from build123d import *

# Parameters (mm, degrees)
SKETCH_R           = 3.5
PAD_DEPTH          = 4
SKETCH001_W        = 5
SKETCH001_H        = 3.5
PAD001_DEPTH       = 17
POLARPATTERN_COUNT = 4
PAD002_DEPTH       = 17
PAD004_DEPTH       = 4
PAD005_DEPTH       = 20


with BuildPart() as part:
    # Sketch → Pad (new body)
    with BuildSketch(Plane.XY):
        Polygon((-9.8, 2.5), (-9.8, -2.5), (-2.5, -9.8), (2.5, -9.8), (9.8, -2.5), (9.8, 2.5), (2.5, 9.8), (-2.5, 9.8), align=None)
        Circle(SKETCH_R, mode=Mode.SUBTRACT)
    extrude(amount=-PAD_DEPTH)

    # Sketch001 → Pad001 (join)
    with BuildSketch(Plane.XY):
        with Locations((0, 8.05)):
            Rectangle(SKETCH001_W, SKETCH001_H)
    pad001 = extrude(amount=PAD001_DEPTH)

    # PolarPattern: Pad001 ×4 about axis
    polarpattern_axis = Axis((0, 0, 0), (0, 0, 1))
    for i in range(1, POLARPATTERN_COUNT):
        add(pad001.rotate(polarpattern_axis, i * 360 / POLARPATTERN_COUNT))

    # Sketch002 → Pad002 (join)
    with BuildSketch(Plane.XY):
        Polygon((-2.5, 9.8), (-5, 54.8), (5, 54.8), (2.5, 9.8), align=None)
    extrude(amount=PAD002_DEPTH)

    # Sketch002 → Pad004 (join)
    with BuildSketch(Plane.XY):
        Polygon((-2.5, 9.8), (-5, 54.8), (5, 54.8), (2.5, 9.8), align=None)
    extrude(amount=-PAD004_DEPTH)

    # Sketch003 → Pad005 (join, symmetric)
    with BuildSketch(Plane.YZ):
        Polygon((51.097133, 17), (95.802441, 17), (95.802441, 13), (55.802441, 13), (60.210616, -12), (56.210616, -12), align=None)
    extrude(amount=PAD005_DEPTH, both=True)


solid = part.part
The listing builds one solid part. Answer for the finished solid, in the listing's coordinates (mm). A direction names the side the tool comes from. Coordinates: 2 decimals unless noted, no trailing zeros. Write each loop counter-clockwise with the first axis right and the second up, starting at its lowest first coordinate (ties: lowest second). Pieces come first, ordered by that corner, then holes. Notation, with made-up numbers: M -37.75,77.5 L -15.75,77.5 A6 ccw -15.75,86.5 Z; hole C 53,-35.75 d4. An arc over 180 degrees is marked long. Write each question's results on one line, items separated by ' | '.
Item 1: Which of the six approach directions +Z, -Z, +X, -X, +Y, -Y give full straight-line access (tool end or side, diameter ignored) to faces 4 (the face through (-2.5, 8, 8)), 5 (the face through (0.28, 57.976, 0.675)), 6 (the face through (8, -2.5, 8))?
Answer below:
face 4: +Z, -X, -Y | face 5: +X, -X, +Y | face 6: +Z, +X, -X, -Y
Item 2: Consider probe 1 along X at (y, z) = (27.5, -3.25); probe 2 along Z at (x, y) = (-13, 91.5); probe 3 along Z at (x, y) = (2, 48). Determine where each line is inside the solid, lowest interval first. Write a range as [from, to].
Answer below:
probe 1: [-3.48, 3.48] | probe 2: [13, 17] | probe 3: [-4, 17]
Item 3: For a pull along Y with two mould halves and no side action, classify faces 1 (the face through (0, 23, -4)), 2 (the face through (3.233, -1.341, -1.972)), 3 (the face through (0, -9.8, 6)) as released by +Y, released by -Y, zero draft, split by the parting line, or undercut.
Answer below:
face 1: zero draft | face 2: undercut | face 3: released by -Y
Item 4: The part is cut by section A-A on y = 0. Determine the outline of the cut face in (x, z).
Answer below:
outline: M -9.8,-4 L -3.5,-4 L -3.5,0 L -6.3,0 L -6.3,17 L -9.8,17 Z; M 3.5,-4 L 9.8,-4 L 9.8,17 L 6.3,17 L 6.3,0 L 3.5,0 Z
Item 5: The part is cut by section B-B on x = 0. Determine the outline of the cut face in (y, z), and give its area (3 significant figures).
Answer below:
outline: M -9.8,-4 L -3.5,-4 L -3.5,0 L -6.3,0 L -6.3,17 L -9.8,17 Z; M 3.5,-4 L 54.8,-4 L 56.21,-12 L 60.21,-12 L 55.8,13 L 95.8,13 L 95.8,17 L 6.3,17 L 6.3,0 L 3.5,0 Z | area: 1,350 mm2
Item 6: The part is cut by section D-D on x = 8. Determine the outline of the cut face in (y, z), and give its area (3 significant figures).
Answer below:
outline: M -4.3,-4 L 4.3,-4 L 4.3,0 L 2.5,0 L 2.5,17 L -2.5,17 L -2.5,0 L -4.3,0 Z; M 51.1,17 L 56.21,-12 L 60.21,-12 L 55.8,13 L 95.8,13 L 95.8,17 Z | area: 397 mm2
Item 7: Given P1, Ø1.8, axis at y = -8, z = 8, coming from the +X side; P2, Ø20, axis at x = -7.5, y = 78.5, coming from the -Z side; P3, Ø3, axis at x = 5.5, z = -7, coming from the +Y side; P4, Ø4, axis at x = -7, y = 42, coming from the -Z side (3 decimals), each flat-ended and moving along its own axis, determine where each tip first touches the part or whether it passes through.
Answer below:
P1: x = 2.5 | P2: z = 13 | P3: y = 59.59 | P4: through
Item 8: The part is cut by section C-C on z = 2.5. Determine the outline of the cut face in (x, y).
Answer below:
outline: M -20,53.65 L -4.94,53.65 L -2.5,9.8 L -2.5,6.3 L 2.5,6.3 L 2.5,9.8 L 4.94,53.65 L 20,53.65 L 20,57.65 L -20,57.65 Z; M -9.8,-2.5 L -6.3,-2.5 L -6.3,2.5 L -9.8,2.5 Z; M -2.5,-9.8 L 2.5,-9.8 L 2.5,-6.3 L -2.5,-6.3 Z; M 6.3,-2.5 L 9.8,-2.5 L 9.8,2.5 L 6.3,2.5 Z
